Here's how the part is built. I have some questions about the finished solid (model axes, mm). A direction names the side the tool comes from. Round coordinates to 2 decimals unless told otherwise and drop trailing zeros. Loops run counter-clockwise (first coordinate to the right, second up) from the corner with the lowest first, then second, coordinate; pieces in that order, holes last. Notation, with made-up numbers: M -34,21.5 L -13,21.5 A19 ccw -13,50.5 Z; hole C -18.5,37 d2. An arc over 180 degrees is marked long. Use a Markdown table: item, result.
```python
from build123d import *

# Parameters (mm, degrees)
SKETCH1_R           = 2.4892
SKETCH1_R_2         = 4.0635
BOSS_EXTRUDE1_DEPTH = 7.62


with BuildPart() as part:
    # Sketch1 → Boss-Extrude1 (new body)
    with BuildSketch(Plane.XY):
        Polygon((0, 12.964410589), (432.660000058, 12.964410589), (432.660000058, 5.019410589), (457.2, 5.019410589), (457.2, -4.800589411), (0, -4.800589411), align=None)
        with Locations(Location((386.08, 4.081910589, 0), (0, 0, 180))):
            Circle(SKETCH1_R, mode=Mode.SUBTRACT)
        with Locations(Location((228.6, 4.081910589, 0), (0, 0, 180))):
            Circle(SKETCH1_R, mode=Mode.SUBTRACT)
        with Locations(Location((71.12, 4.081910589, 0), (0, 0, 180))):
            Circle(SKETCH1_R, mode=Mode.SUBTRACT)
        with Locations(Location((13.54, 2.599410589, 0), (0, 0, 180))):
            Circle(SKETCH1_R_2, mode=Mode.SUBTRACT)
    extrude(amount=BOSS_EXTRUDE1_DEPTH)


solid = part.part
```
Q1. For faces 1 (the flat face through (232, 4, 0)), 2 (the flat face through (432.66, 9, 4)), which set-ups out of +Z, -Z, +X, -X, +Y, -Y let a thin tool reach every point of the face, with its end or its side?
Return value:
| item | result |
|---|---|
| face 1 | -Z, +X, -X, +Y, -Y |
| face 2 | +Z, -Z, +X, +Y |
Q2. Imagine slicing it at A-A, the plane x = 13.54. Please give me the cut outline in (y, z), then the cut area to 3 significant figures.
Return value:
| item | result |
|---|---|
| outline | M -4.8,0 L -1.46,0 L -1.46,7.62 L -4.8,7.62 Z; M 6.66,0 L 12.96,0 L 12.96,7.62 L 6.66,7.62 Z |
| area | 73.4 mm^2 |
Q3. I need wall thicknesses on line 1 (Y direction, x = 71.12, z = 4.25); line 2 (X direction, y = 2.75, z = 2.75); line 3 (Y direction, x = 13.54, z = 4.5). Which ranges of each line are inside material? Lowest first, please. Write a range as from..to.
Return value:
| item | result |
|---|---|
| line 1 | y = -4.8..1.59, 6.57..12.96 |
| line 2 | x = 0..9.48, 17.6..69.02, 73.22..226.5, 230.7..383.98, 388.18..457.2 |
| line 3 | y = -4.8..-1.46, 6.66..12.96 |
Q4. We'd pull the mould along Y, two halves only. Please class faces 3 (the flat face through (445, 5.019, 4)), 4 (the flat face through (232, -4.801, 4)), 5 (the flat face through (457.2, 0, 4)), 6 (the cylindrical face through (9.664, 1.379, 3.757)): pulls with the +Y half, pulls with the -Y half, needs draft (parallel to the pull), parting line crosses it, or undercut.
Return value:
| item | result |
|---|---|
| face 3 | pulls with the +Y half |
| face 4 | pulls with the -Y half |
| face 5 | needs draft |
| face 6 | undercut |
Q5. Imagine slicing it at B-B, the plane z = 4.5. Please give me the cut outline in (x, y), then the cut area to 3 significant figures.
Return value:
| item | result |
|---|---|
| outline | M 0,-4.8 L 457.2,-4.8 L 457.2,5.02 L 432.66,5.02 L 432.66,12.96 L 0,12.96 Z; hole C 13.54,2.6 d8.13; hole C 71.12,4.08 d4.98; hole C 228.6,4.08 d4.98; hole C 386.08,4.08 d4.98 |
| area | 7,820 mm^2 |
Q6. Will this pin go through, and if not, where does the flat tip stop? P1, Ø4, axis at x = 441.5, z = 3, coming from the +Y side.
Return value:
| item | result |
|---|---|
| P1 | stops at y = 5.02 |
